Geometry check sheet. Reference: drawing and pictorial views, mm from the part's lowest x, y, z. A direction names the side the tool comes from. Coordinates: 2 decimals unless noted, no trailing zeros. Loops run counter-clockwise (first coordinate to the right, second up) from the corner with the lowest first, then second, coordinate; pieces in that order, holes last. Notation, with made-up numbers: M 27.5,26 L 49.5,26 A26 ccw 49.5,51 Z; hole C 4,27.5 d7. An arc over 180 degrees is marked long. Write each question's results on one line, items separated by ' | '. Start each with the question number.
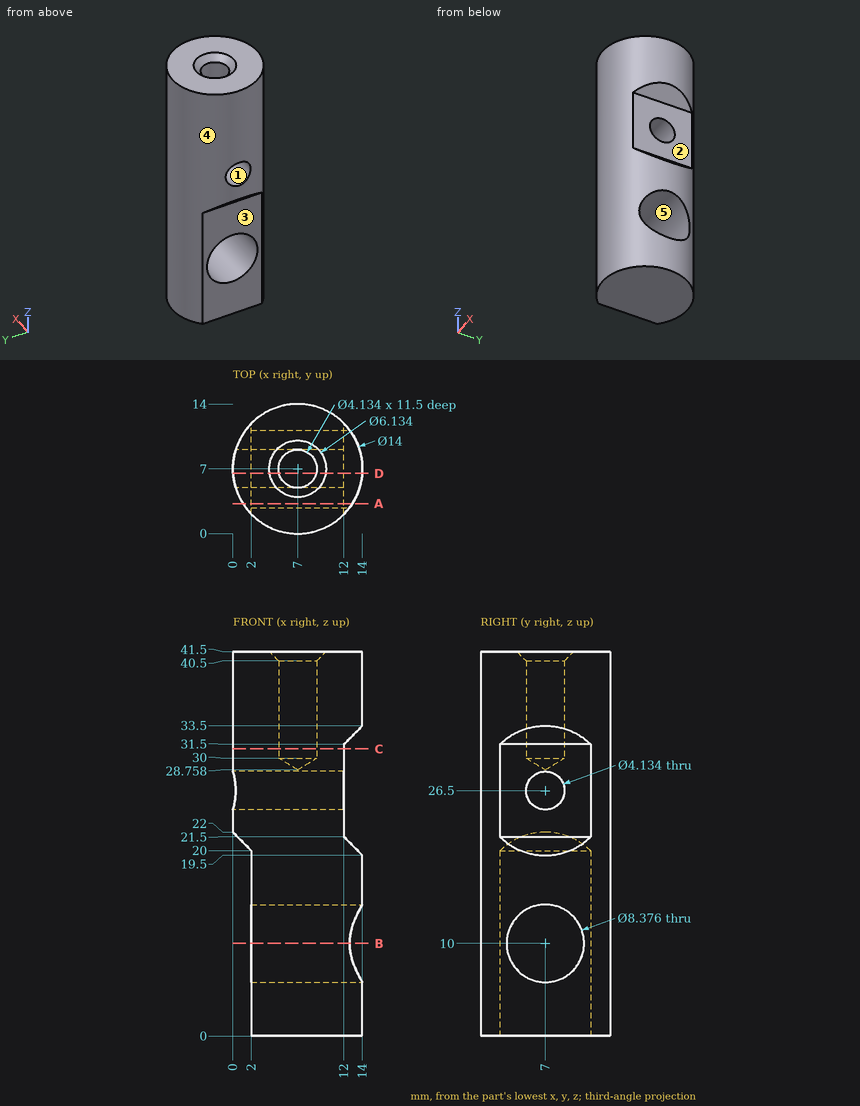
1) Thickness scan on probe 1 along Y at (x, z) = (7.5, 31.5); probe 2 along X at (y, z) = (12, 32); probe 3 along X at (y, z) = (7, 33). Record the ranges inside material, lowest first.
2) Section check C-C (z = 31). Enter the section's corners in (x, y), then the cut area to 3 significant figures.
3) Section check B-B (z = 10). Enter the section's corners in (x, y).
4) Gauge pin test, flat ends, axial feed: P1, Ø4, axis at x = 11.5, z = 8.5, coming from the +Y side; P2, Ø4, axis at x = 2, z = 35.5, coming from the +Y side; P3, Ø3, axis at y = 6.5, z = 14, coming from the -X side. Record the tip position at first contact, or that the pin passes through.
5) Set-up check for the marked faces 1 and 2: record each of +Z, -Z, +X, -X, +Y, -Y from which the full face is reachable in a straight line by a thin tool's end or side.
6) Section check D-D (y = 6.5). Give the number of separate pieces and of enclosed holes in the cut face, then the cut area to 3 significant figures.
7) Release check for a two-part mould opening along Y. For the marked faces 3, 4 and 5 record: +Y half, -Y half, draft (parallel to the pull), parting line (faces both ways), or undercut.
8) Section check A-A (y = 3.25). Enter the section's corners in (x, z), then the cut area to 3 significant figures.
Return value:
1) probe 1: y = 0.02 to 4.99, 9.01 to 13.98 | probe 2: x = 2.1 to 11.9 | probe 3: x = 0 to 4.93, 9.07 to 13.5
2) outline: M 12,2.1 L 12,11.9 A7 ccw long Z; hole C 7,7 d4.13 | area: 127 mm2
3) outline: M 2,2.1 A7 ccw 12.61,2.81 L 2,2.81 Z; M 2,11.19 L 12.61,11.19 A7 ccw 2,11.9 Z
4) P1: stops at y = 13.54 | P2: stops at y = 13.32 | P3: stops at x = 2
5) face 1: +X, -X | face 2: +X, +Y, -Y
6) separate pieces: 3 | enclosed holes: 0 | area: 317 mm2
7) face 3: draft | face 4: parting line | face 5: undercut
8) outline: M 1.09,20.91 L 2,20 L 2,11.86 L 12.91,11.86 L 12.91,20.59 L 12,21.5 L 12,31.5 L 12.91,32.41 L 12.91,41.5 L 1.09,41.5 Z; M 2,0 L 12.91,0 L 12.91,8.14 L 2,8.14 Z | area: 421 mm2
